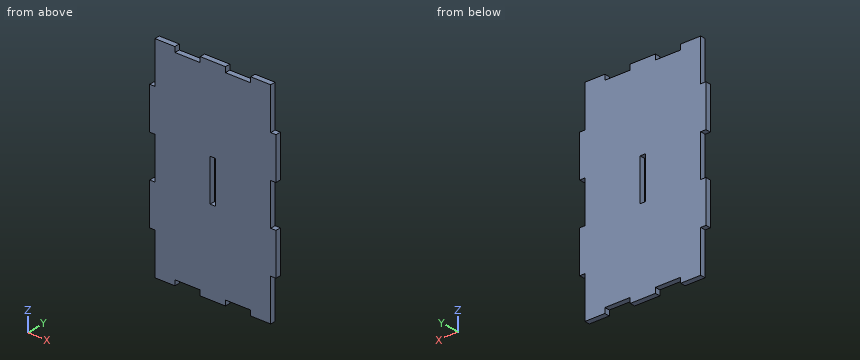
from build123d import *

# Parameters (mm, degrees)
SKETCH1_W           = 76.2
SKETCH1_H           = 127
BOSS_EXTRUDE1_DEPTH = 3.175
SKETCH2_W           = 3.175
SKETCH2_H           = 25.4
CUT_EXTRUDE1_DEPTH  = 3.175
LPATTERN1_COUNT     = 3
LPATTERN1_PITCH     = 50.8
SKETCH3_W           = 15.24
SKETCH3_H           = 3.175
CUT_EXTRUDE2_DEPTH  = 3.175
LPATTERN2_COUNT     = 3
LPATTERN2_PITCH     = 30.48
SKETCH4_W           = 3.175
SKETCH4_H           = 25.4
CUT_EXTRUDE3_DEPTH  = 3.175


with BuildPart() as part:
    # Sketch1 → Boss-Extrude1 (new body)
    with BuildSketch(Plane(origin=(0, 0, 0), x_dir=(1, 0, 0), z_dir=(0, 1, 0))):
        Rectangle(SKETCH1_W, SKETCH1_H)
    extrude(amount=BOSS_EXTRUDE1_DEPTH)

    # Sketch2 → Cut-Extrude1 (cut)
    with BuildSketch(Plane(origin=(0, 3.175, 0), x_dir=(1, 0, 0), z_dir=(0, 1, 0))):
        with Locations((-36.5125, 50.8)):
            Rectangle(SKETCH2_W, SKETCH2_H)
        with Locations((36.5125, 50.8)):
            Rectangle(SKETCH2_W, SKETCH2_H)
    cut_extrude1 = extrude(amount=-CUT_EXTRUDE1_DEPTH, mode=Mode.SUBTRACT)

    # LPattern1: Cut-Extrude1 ×3
    with Locations(*[(0, 0, i * LPATTERN1_PITCH) for i in range(1, LPATTERN1_COUNT)]):
        add(cut_extrude1, mode=Mode.SUBTRACT)

    # Sketch3 → Cut-Extrude2 (cut)
    with BuildSketch(Plane(origin=(0, 3.175, 0), x_dir=(1, 0, 0), z_dir=(0, 1, 0))):
        with Locations((15.24, 61.9125)):
            Rectangle(SKETCH3_W, SKETCH3_H)
        with Locations((15.24, -61.9125)):
            Rectangle(SKETCH3_W, SKETCH3_H)
    cut_extrude2 = extrude(amount=-CUT_EXTRUDE2_DEPTH, mode=Mode.SUBTRACT)

    # LPattern2: Cut-Extrude2 ×3
    with Locations(*[(-i * LPATTERN2_PITCH, 0, 0) for i in range(1, LPATTERN2_COUNT)]):
        add(cut_extrude2, mode=Mode.SUBTRACT)

    # Sketch4 → Cut-Extrude3 (cut)
    with BuildSketch(Plane(origin=(0, 3.175, 0), x_dir=(1, 0, 0), z_dir=(0, 1, 0))):
        Rectangle(SKETCH4_W, SKETCH4_H)
    extrude(amount=-CUT_EXTRUDE3_DEPTH, mode=Mode.SUBTRACT)


solid = part.part
Geometry check sheet. Reference: the model listing, model coordinates, mm. Give positions to 0.01 mm unless a question says otherwise; leave off trailing zeros. Loops run counter-clockwise (first coordinate to the right, second up) from the corner with the lowest first, then second, coordinate; pieces in that order, holes last. Notation, with made-up numbers: M 69.25,1 L 97.25,1 A29 cw 97.25,38 Z; hole C 29,-29 d11. An arc over 180 degrees is marked long. Write each question's results on one line, items separated by ' | '.
1) Thickness scan on line 1 (X direction, y = 0.5, z = 1) (1 decimal); line 2 (X direction, y = 0.85, z = 50) (3 decimals); line 3 (Z direction, x = -22.5, y = 3) (3 decimals). Record the ranges inside material, lowest first.
Answers follow:
line 1: -34.9 to -1.6, 1.6 to 34.9 | line 2: -34.925 to 34.925 | line 3: -60.325 to 60.325
2) Gauge pin test, flat ends, axial feed: pin 1 (1 mm diameter, centred on x = -15, y = 1.5, fed in from -Z) (3 decimals); pin 2 (1 mm diameter, centred on y = 2, z = 62.5, fed in from -X) (3 decimals); pin 3 (1.6 mm diameter, centred on y = 1, z = 54, fed in from +X) (3 decimals). Record the tip position at first contact, or that the pin passes through.
Answers follow:
pin 1: z = -60.325 | pin 2: x = -34.925 | pin 3: x = 34.925
3) Section check A-A, the plane z = -5. Record the boundary of the cut face in (x, y) (1 decimal).
Answers follow:
outline: M -34.9,0 L -1.6,0 L -1.6,3.2 L -34.9,3.2 Z; M 1.6,0 L 34.9,0 L 34.9,3.2 L 1.6,3.2 Z
4) Section check C-C, the plane z = 40.5. Record the boundary of the cut face in (x, y) (3 decimals).
Answers follow:
outline: M -34.925,0 L 34.925,0 L 34.925,3.175 L -34.925,3.175 Z
5) Section check B-B, the plane x = -19.5. Record the boundary of the cut face in (y, z) (3 decimals), plus the area to 3 significant figures.
Answers follow:
outline: M 0,-60.325 L 3.175,-60.325 L 3.175,60.325 L 0,60.325 Z | area: 383 mm2
